```python
from build123d import *

# Parameters (mm, degrees)
F1_DEPTH = 2
F2_DEPTH = 13
F3_R     = 1


with BuildPart() as f1:
    # F0 (on Top) → F1 (new body)
    with BuildSketch(Plane.XY):
        Polygon((0, 0), (0, 20.581139), (-9.5, 23.747805), (-9.5, 0), align=None)
        Polygon((-1.5, 1.5), (-7.5, 1.5), (-7.5, 21.5), (-1.5, 19.5), align=None, mode=Mode.SUBTRACT)
        Polygon((-7.5, 21.5), (-7.5, 1.5), (-1.5, 1.5), (-1.5, 19.5), align=None)
    extrude(amount=F1_DEPTH)

    # F0 (on Top) → F2 (join)
    with BuildSketch(Plane.XY):
        Polygon((-7.5, 21.5), (-7.5, 1.5), (-1.5, 1.5), (-1.5, 19.5), align=None)
    extrude(amount=F2_DEPTH)

    # F3
    f3_edges = [f1.edges().sort_by_distance(p)[0] for p in [
        (-7.5, 21.5, 7.5),
        (-9.5, 23.747805, 1),
        (0, 20.581139, 1),
        (-1.5, 19.5, 7.5),
        (0, 0, 1),
        (-1.5, 1.5, 7.5),
        (-9.5, 0, 1),
        (-7.5, 1.5, 7.5),
        (-9.5, 11.873903, 0),
        (-4.75, 0, 0),
        (-4.75, 22.164472, 0),
        (0, 10.290569, 0),
    ]]
    fillet(f3_edges, radius=F3_R)


solid = f1.part
```
Verification items for the finished model (mm, model axes). A direction names the side the tool comes from. Give positions to 0.01 mm unless a question says otherwise; leave off trailing zeros. Order: outer loops, then holes, each group sorted by start corner. A loop starts at its lowest first (then second) coordinate and runs counter-clockwise, first axis right, second up. Notation, with made-up numbers: M 70.25,-7 L 117.25,-7 A11 cw 117.25,12 Z; hole C 52,-20.5 d3. An arc over 180 degrees is marked long. Return JSON: item names as keys, results as strings. Group by question number.
1) Section check C-C on x = -9. Record the cut outline in (y, z), and give its area (3 significant figures).
2) Scan lines: line 1 (Z direction, x = -8.25, y = 9.25); line 2 (X direction, y = 6, z = 9.5); line 3 (Y direction, x = -7.25, z = 6.5). Record each from-to range of solid material in increasing order.
3) Section check D-D on y = 19.25. Record the cut outline in (x, z).
4) Go/stop test with flat-tipped pins: pin 1 Ø2 at (x, z) = (-5, 6) entering from +Y; pin 2 Ø5.5 at (y, z) = (12, 7.5) entering from -X; pin 3 Ø2 at (x, z) = (-4, 4) entering from -Y. Record where each tip stops, or that it passes through.
5) Section check B-B on y = 9.75. Record the cut outline in (x, z), and give its area (3 significant figures).
6) Section check A-A on z = 4. Record the cut outline in (x, y), and give its area (3 significant figures).
7) Access from +Z, -Z, +X, -X, +Y, -Y to the whole of each face (thin tool, end or side, straight path). Record for faces 1 (the face through (-7.074, 20.931, 7.577)), 2 (the face through (-4.2, 20.4, 7.4)), 3 (the face through (-1.5, 11, 7)).
Answer block:
{
 "1": {"outline": "M 0.13,1 A0.87 ccw 1,0.13 L 22.36,0.13 A0.87 ccw 23.23,1 L 23.23,2 L 0.13,2 Z", "area": "42.8 mm^2"},
 "2": {"line 1": "z = 0 to 2", "line 2": "x = -7.5 to -1.5", "line 3": "y = 1.84 to 20.77"},
 "3": {"outline": "M -9.5,1 A1 ccw -8.5,0 L -1,0 A1 ccw 0,1 L 0,2 L -1.62,2 L -1.62,13 L -7.5,13 L -7.5,2 L -9.5,2 Z"},
 "4": {"pin 1": "stops at y = 21", "pin 2": "stops at x = -7.5", "pin 3": "stops at y = 1.5"},
 "5": {"outline": "M -9.5,1 A1 ccw -8.5,0 L -1,0 A1 ccw 0,1 L 0,2 L -1.5,2 L -1.5,13 L -7.5,13 L -7.5,2 L -9.5,2 Z", "area": "84.6 mm^2"},
 "6": {"outline": "M -7.5,2.5 A1 ccw -6.5,1.5 L -2.5,1.5 A1 ccw -1.5,2.5 L -1.5,18.78 A1 ccw -2.18,19.73 L -6.18,21.06 A1 ccw -7.5,20.11 Z", "area": "113 mm^2"},
 "7": {"face 1": "+Z, +Y", "face 2": "+Z, +X, +Y", "face 3": "+Z, +X, +Y, -Y"}
}
